The model under review builds one solid part; all positions refer to its coordinate system, in mm. Face numbers are marked on the shaded views. A direction names the side the tool comes from. Give positions to 0.01 mm unless a question says otherwise; leave off trailing zeros. Write each loop counter-clockwise with the first axis right and the second up, starting at its lowest first coordinate (ties: lowest second). Pieces come first, ordered by that corner, then holes. Notation, with made-up numbers: (48, 18) - (85, 18) arc R13 cw to (85, 27) - close; hole circle Ø11 at (87, -2.5). An arc over 180 degrees is marked (long way). Write item = value, one per line.
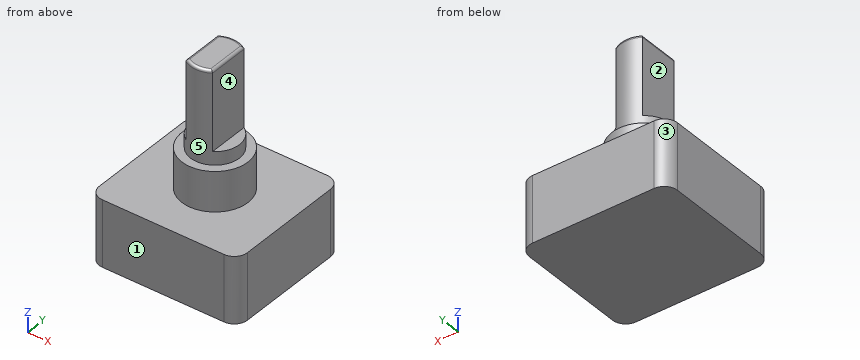
Autodesk Inventor part; units mm, degrees
ref_plane "РабПлоскость1" through (0, 0, 8) normal (0, 0, 1) x (1, 0, 0)
ref_plane "YZ Plane" through (0, 0, 0) normal (1, 0, 0) x (0, 1, 0)
ref_plane "XZ Plane" through (0, 0, 0) normal (0, 1, 0) x (-1, 0, 0)
sketch "Эскиз1" plane through (0, 0, 0) normal (0, 0, 1) x (1, 0, 0)
  line L0 (-5.6, 5.1) -> (5.6, 5.1)
  line L1 (5.6, 5.1) -> (5.6, -5.1)
  line L2 (5.6, -5.1) -> (-5.6, -5.1)
  line L3 (-5.6, -5.1) -> (-5.6, 5.1)
  line L4 (-5.6, 5.1) -> (5.6, -5.1) construction
  line L5 (5.6, 5.1) -> (-5.6, -5.1) construction
  point P0 (0, 0)
  dimension "d0" = 11.2
  dimension "d1" = 10.2
extrude "Выдавливание1" add sketch "Эскиз1" along normal blind 5
fillet "Сопряжение1" radius 1 4 edges at (-5.6, 5.1, 2.5) (5.6, 5.1, 2.5) (5.6, -5.1, 2.5) (-5.6, -5.1, 2.5)
sketch "Эскиз2" plane through (0, 0, 5) normal (0, 0, 1) x (1, 0, 0)
  circle A0 centre (0, 0) radius 2.5
  dimension "d5" = 5
extrude "Выдавливание2" add sketch "Эскиз2" along normal blind 3
sketch "Эскиз3" plane through (0, 0, 8) normal (0, 0, 1) x (1, 0, 0)
  circle A0 centre (0, 0) radius 1.85
  dimension "d8" = 3.7
extrude "Выдавливание3" add sketch "Эскиз3" along normal blind 7
sketch "Эскиз4" plane through (0, 0, 15) normal (0, 0, 1) x (1, 0, 0)
  line L0 (1, -5) -> (-1, -5)
  line L1 (-1, -5) -> (-1, 5)
  line L2 (-1, 5) -> (1, 5)
  line L3 (1, 5) -> (1, -5)
  line L4 (1, -5) -> (-1, 5) construction
  line L5 (-1, -5) -> (1, 5) construction
  line L6 (-1, 5) -> (-9.7743, 5)
  line L7 (-9.7743, 5) -> (-9.7743, -5)
  line L8 (-9.7743, -5) -> (-1, -5)
  line L9 (-1, -5) -> (-1, 5)
  line L10 (1, -5) -> (12.6944, -5)
  line L11 (12.6944, -5) -> (12.6944, 8.8009)
  line L12 (12.6944, 8.8009) -> (1, 8.8009)
  line L13 (1, 8.8009) -> (1, -5)
  point P0 (0, 0)
  dimension "d11" = 2
  dimension "d12" = 10
extrude "Выдавливание4" cut sketch "Эскиз4" against normal blind 6 contours L3 L13 L12 L11 L10 | L8 L7 L6 L1
fillet "Сопряжение2" radius 0.2 4 edges at (0, -1.85, 15) (0, 1.85, 15) (1, 0, 15) (-1, 0, 15)
ref_plane "РабПлоскость1" through (0, 0, 8) normal (0, 0, 1) x (1, 0, 0)
properties part number "Потенциометр"
1. Take a section at B-B on y = -0.5. Give the boundary of the cut face in (x, z).
Findings below:
outline = (-5.6, 0) - (5.6, 0) - (5.6, 5) - (2.45, 5) - (2.45, 8) - (1.78, 8) - (1.78, 9) - (1, 9) - (1, 14.8) arc R0.2 ccw to (0.8, 15) - (-0.8, 15) arc R0.2 ccw to (-1, 14.8) - (-1, 9) - (-1.78, 9) - (-1.78, 8) - (-2.45, 8) - (-2.45, 5) - (-5.6, 5) - close
2. Take a section at A-A on x = -1.5. Give the boundary of the cut face in (y, z), and give its area (3 significant figures).
Findings below:
outline = (-5.1, 0) - (5.1, 0) - (5.1, 5) - (2, 5) - (2, 8) - (1.08, 8) - (1.08, 9) - (-1.08, 9) - (-1.08, 8) - (-2, 8) - (-2, 5) - (-5.1, 5) - close
area = 65.2 mm²
3. For line 1 (Z direction, x = -0.25, y = 3.75); line 2 (X direction, y = -0.25, z = 13); line 3 (X direction, y = 4.5, z = 3.25), list the stretches that pass through material, from the lowest coordinate up. Write a range as from..to.
Findings below:
line_1 = 0..5
line_2 = -1..1
line_3 = -5.52..5.52
4. Take a section at D-D on x = 0. Give the boundary of the cut face in (y, z), and give its area (3 significant figures).
Findings below:
outline = (-5.1, 0) - (5.1, 0) - (5.1, 5) - (2.5, 5) - (2.5, 8) - (1.85, 8) - (1.85, 14.8) arc R0.2 ccw to (1.65, 15) - (-1.65, 15) arc R0.2 ccw to (-1.85, 14.8) - (-1.85, 8) - (-2.5, 8) - (-2.5, 5) - (-5.1, 5) - close
area = 91.9 mm²
5. Insertion check: P1, Ø0.9, axis at x = -1.5, y = -0.5, coming from the +Z side; P2, Ø0.9, axis at y = -1, z = 11, coming from the +X side; P3, Ø1.6, axis at y = 0.5, z = 11.5, coming from the -X side. Each pin has a flat end and moves straight along its axis. Give the tip position at first contact, or say it passes through.
Findings below:
P1 = 9
P2 = 1
P3 = -1
6. Take a section at C-C on z = 7. Give the boundary of the cut face in (x, y).
Findings below:
outline = circle Ø5 at (0, 0)
7. Machinability: for the marked faces 1, 2, 3, 4 and 5, which of the approach directions +Z, -Z, +X, -X, +Y, -Y give a long, thin tool a straight path to every point of the face, cutting with its end or side? Answer none if there is none.
Findings below:
face_1 = +Z, -Z, +X, -X, -Y
face_2 = +Z, -X, +Y, -Y
face_3 = +Z, -Z, -X, +Y
face_4 = +Z, +X, +Y, -Y
face_5 = +Z
